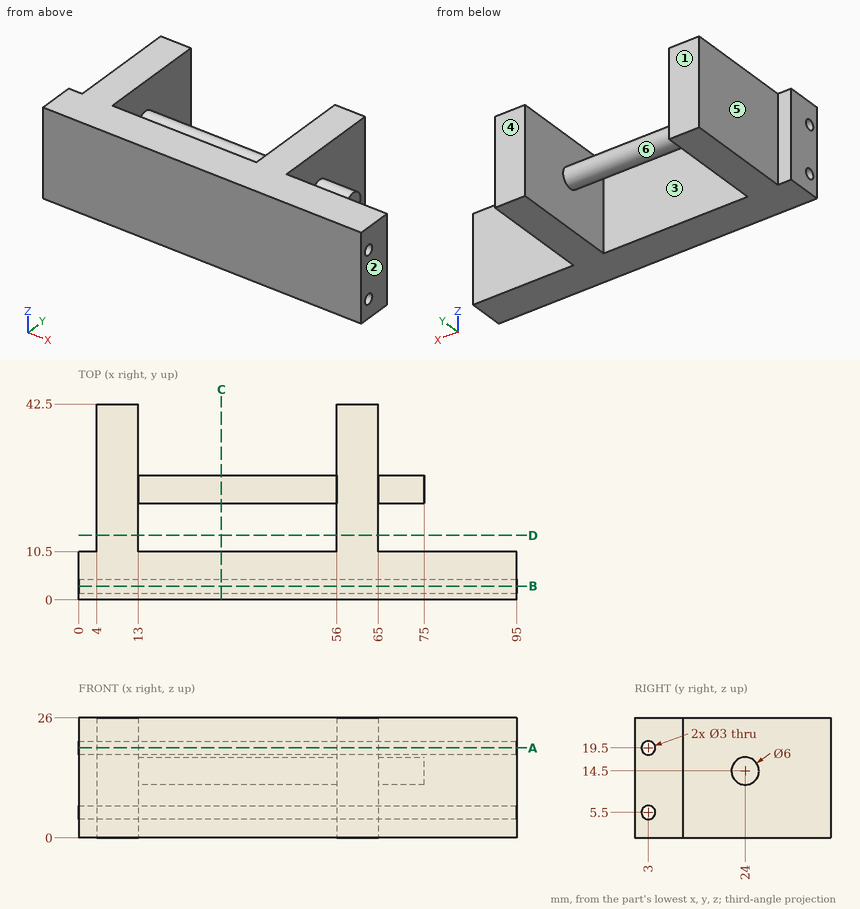
Geometry: see drawing. Coordinates: mm, zero at the bounding-box minimum. A direction names the side the tool comes from. Give positions to 0.01 mm unless a question says otherwise; leave off trailing zeros. Loops run counter-clockwise (first coordinate to the right, second up) from the corner with the lowest first, then second, coordinate; pieces in that order, holes last. Notation, with made-up numbers: (2.25, 46.25) -> (60.25, 46.25) arc R16 cw to (60.25, 77.25) -> close; hole circle Ø9 at (-36, 44). An arc over 180 degrees is marked (long way). Put each result on its own line as item: value.
1. Set-up query: the marked faces 4, 5 and 6. Return all of +Z, -Z, +X, -X, +Y, -Y with unobstructed straight access to the full face (end or side cutting, diameter ignored); none if empty.
Taken from the geometry:
face 4: +Z, -Z, +X, -X, +Y
face 5: +Z, -Z, -X, +Y
face 6: none
2. Pull-direction query (X, two-part tool) for the marked faces 1, 2 and 3; classes: released by +X, released by -X, zero draft, split by the parting line, or undercut.
Taken from the geometry:
face 1: zero draft
face 2: released by +X
face 3: undercut
3. Ray query, line 1 along X through (y, z) = (33, 22.5); line 2 along Z through (x, y) = (68, 2); line 3 along Y through (x, z) = (59, 19.5). Return the intervals inside material, ascending. Write a range as [from, to].
Taken from the geometry:
line 1: x = [4, 13], [56, 65]
line 2: z = [0, 4.38], [6.62, 18.38], [20.62, 26]
line 3: y = [0, 1.5], [4.5, 42.5]
4. Cut plane A-A (z = 19.5). Return the cut outline in (x, y), plus the area to 3 significant figures.
Taken from the geometry:
outline: (0, 0) -> (95, 0) -> (95, 1.5) -> (0, 1.5) -> close; (0, 4.5) -> (95, 4.5) -> (95, 10.5) -> (65, 10.5) -> (65, 42.5) -> (56, 42.5) -> (56, 10.5) -> (13, 10.5) -> (13, 42.5) -> (4, 42.5) -> (4, 10.5) -> (0, 10.5) -> close
area: 1,290 mm2
5. Pin query (flat end, axial travel): P1, Ø8, axis at y = 26, z = 7, coming from the +X side; P2, Ø8, axis at y = 33.5, z = 17.5, coming from the -X side; P3, Ø3, axis at x = 2, z = 15.5, coming from the +Y side. Return the tip coordinate at first contact, or that it passes through.
Taken from the geometry:
P1: stops at x = 65
P2: stops at x = 4
P3: stops at y = 10.5
6. Cut plane B-B (y = 3). Return the cut outline in (x, z).
Taken from the geometry:
outline: (0, 0) -> (95, 0) -> (95, 4) -> (0, 4) -> close; (0, 7) -> (95, 7) -> (95, 18) -> (0, 18) -> close; (0, 21) -> (95, 21) -> (95, 26) -> (0, 26) -> close
7. Cut plane D-D (y = 14). Return the cut outline in (x, z), plus the area to 3 significant figures.
Taken from the geometry:
outline: (4, 0) -> (13, 0) -> (13, 26) -> (4, 26) -> close; (56, 0) -> (65, 0) -> (65, 26) -> (56, 26) -> close
area: 468 mm2
8. Cut plane C-C (x = 31). Return the cut outline in (y, z).
Taken from the geometry:
outline: (0, 0) -> (10.5, 0) -> (10.5, 26) -> (0, 26) -> close; circle Ø6 at (24, 14.5); hole circle Ø3 at (3, 5.5); hole circle Ø3 at (3, 19.5)
